Source: CAD feature listing. Evaluate the final solid. Frame: model axes, mm. A direction names the side the tool comes from. Give positions to 0.01 mm unless a question says otherwise; leave off trailing zeros. Write each loop counter-clockwise with the first axis right and the second up, starting at its lowest first coordinate (ties: lowest second). Pieces come first, ordered by that corner, then holes. Notation, with made-up numbers: (16, 71) -> (29, 71) arc R34 ccw to (29, 106) -> close; hole circle Ø3 at (84.25, -39.75). An arc over 180 degrees is marked (long way). Answer as a JSON object with one key per item and string values. Group by question number.
Item 1: Section query D-D on x = 70.5. Return the cut outline in (y, z).
Item 2: Section query A-A on y = 15. Return the cut outline in (x, z), plus the area to 3 significant figures.
Item 3: Access query for faces 5 (the face through (100, 5, 3)), 6 (the face through (30, 25, 2)). Directions: +Z, -Z, +X, -X, +Y, -Y. A direction counts if a zero-diameter tool reaches every point of the face in a straight line with its end or side. Return the directions, or none.
Item 4: Pull-direction query (Y, two-part tool) for faces 1 (the face through (127.538, 13.085, 2.465)), 2 (the face through (46.835, 10.119, 2.465)), 3 (the face through (80, -15, 3)), 4 (the face through (60, 5, 3)); classes: pulls with the +Y half, pulls with the -Y half, needs draft (parallel to the pull), parting line crosses it, or undercut.
Item 5: Ray query, probe 1 along X at (y, z) = (17, 1.95); probe 2 along Y at (x, z) = (71, 1.8); probe 3 along X at (y, z) = (21, 1.6). Return the intervals inside material, ascending. Write a range as from..to.
Item 6: First-contact query: pin 1 Ø1.5 at (y, z) = (12.5, 3) entering from +X; pin 2 Ø1.5 at (y, z) = (-7.5, 3.5) entering from +X; pin 3 Ø2.5 at (x, z) = (88, 3) entering from +Y; pin 4 Ø6 at (x, y) = (47.92, 15) entering from +Z (3 decimals). Flat tips, straight axial feed; report the tip coordinate or a pass-through.
Item 7: Section query B-B on z = 3.35. Return the cut outline in (x, y).
Item 8: Section query C-C on y = 0. Return the cut outline in (x, z).
from build123d import *

# Parameters (mm, degrees)
ESQUISSE1_R             = 5
BOSS_EXTRU_1_DEPTH      = 5
ESQUISSE2_W             = 40
ESQUISSE2_H             = 40
ENL_V_MAT_EXTRU_1_DEPTH = 5


with BuildPart() as part:
    # Esquisse1 → Boss.-Extru.1 (new body)
    with BuildSketch(Plane.XY):
        with BuildLine():
            Line((0, 25), (160, 25))
            ThreePointArc((160, 25), (185, 0), (160, -25))
            Line((160, -25), (0, -25))
            ThreePointArc((0, -25), (-25, 0), (0, 25))
        make_face()
        with Locations((122.919007565, 15)):
            Circle(ESQUISSE1_R, mode=Mode.SUBTRACT)
        with Locations((47.919007565, 15)):
            Circle(ESQUISSE1_R, mode=Mode.SUBTRACT)
    extrude(amount=BOSS_EXTRU_1_DEPTH)

    # Esquisse2 → Enlèv. mat.-Extru.1 (cut)
    with BuildSketch(Plane.XY.offset(5)):
        with Locations((80, 5)):
            Rectangle(ESQUISSE2_W, ESQUISSE2_H)
    extrude(amount=-ENL_V_MAT_EXTRU_1_DEPTH, mode=Mode.SUBTRACT)


solid = part.part
Worked answers:
{
 "1": {"outline": "(-25, 0) -> (-15, 0) -> (-15, 5) -> (-25, 5) -> close"},
 "2": {"outline": "(-20, 0) -> (42.92, 0) -> (42.92, 5) -> (-20, 5) -> close; (52.92, 0) -> (60, 0) -> (60, 5) -> (52.92, 5) -> close; (100, 0) -> (117.92, 0) -> (117.92, 5) -> (100, 5) -> close; (127.92, 0) -> (180, 0) -> (180, 5) -> (127.92, 5) -> close", "area": "700 mm^2"},
 "3": {"face 5": "+Z, -Z, +Y", "face 6": "+Z, -Z, +X, -X, +Y"},
 "4": {"face 1": "undercut", "face 2": "undercut", "face 3": "pulls with the +Y half", "face 4": "needs draft"},
 "5": {"probe 1": "-18.33..43.34, 52.5..60, 100..118.34, 127.5..178.33", "probe 2": "-25..-15", "probe 3": "-13.56..60, 100..173.56"},
 "6": {"pin 1": "x = 182.07", "pin 2": "x = 184.07", "pin 3": "y = -15", "pin 4": "through"},
 "7": {"outline": "(0, -25) -> (160, -25) arc R25 ccw to (160, 25) -> (100, 25) -> (100, -15) -> (60, -15) -> (60, 25) -> (0, 25) arc R25 ccw to start; hole circle Ø10 at (47.92, 15); hole circle Ø10 at (122.92, 15)"},
 "8": {"outline": "(-25, 0) -> (60, 0) -> (60, 5) -> (-25, 5) -> close; (100, 0) -> (185, 0) -> (185, 5) -> (100, 5) -> close"}
}
